Geometry: final body of the model. Coordinates: model frame, mm. Round coordinates to 2 decimals unless told otherwise and drop trailing zeros. Order: outer loops, then holes, each group sorted by start corner. A loop starts at its lowest first (then second) coordinate and runs counter-clockwise, first axis right, second up. Notation, with made-up numbers: (89, 33.25) - (127, 33.25) arc R7 cw to (127, 37.25) - close; hole circle Ø2 at (69.25, 2.25). An arc over 180 degrees is marked (long way). Put each result on its own line as item: value. Start each with the question number.
(1) Section C-C (x = -66). Output: boundary loops of the cut face in (y, z), and give its area (3 significant figures).
(2) Pin query (flat end, axial travel): P1, Ø23.5, axis at x = -187.38, y = 187.38, coming from the +Z side. Return the tip coordinate at first contact, or that it passes through.
(3) Material intervals for L1, parallel to X at y = -196, z = 0.5; L2, parallel to X at y = -91.5, z = 0.1; L3, parallel to Y at x = -7.5, z = 1.6, sorted ascending. Write a range as [from, to].
(4) Section A-A (y = 0). Output: boundary loops of the cut face in (x, z).
(5) Section D-D (y = 70). Output: boundary loops of the cut face in (x, z).
Autodesk Inventor part; units mm, degrees
ref_plane "YZ Plane" through (0, 0, 0) normal (1, 0, 0) x (0, 1, 0)
ref_plane "XZ Plane" through (0, 0, 0) normal (0, 1, 0) x (-1, 0, 0)
ref_plane "XY Plane" through (0, 0, 0) normal (0, 0, 1) x (1, 0, 0)
sketch "Эскиз1" plane through (0, 0, 0) normal (0, 0, 1) x (1, 0, 0)
  circle A0 centre (0, 0) radius 240
  circle A1 centre (0, 0) radius 290
  dimension "d0" = 480
  dimension "d1" = 580
extrude "Выдавливание1" add sketch "Эскиз1" along normal blind 2
sketch "Эскиз2" plane through (0, 0, 2) normal (0, 0, 1) x (1, 0, 0)
  circle A0 centre (0, 0) radius 290
  line L0 (0, 290) -> (0, 265)
  dimension "d4" = 25
hole "Отверстие1" at (0, 265, 2) direction (0, 0, -1) diameter 26 end through all
pattern_circular "Круговой массив1" count 16 over 360 about axis through (0, 0, -10) along (0, 0, 1) of "Отверстие1"
properties part number "Прокладка крышек цилиндра"
Checks:
1. outline: (-282.39, 0) - (-230.75, 0) - (-230.75, 2) - (-282.39, 2) - close; (230.75, 0) - (282.39, 0) - (282.39, 2) - (230.75, 2) - close
1. area: 207 mm²
2. P1: passes through
3. L1: x = [-213.74, -197.12], [-177.65, -138.51], [138.51, 177.65], [197.12, 213.74]
3. L2: x = [-275.19, -253.24], [-236.42, -221.87], [221.87, 236.42], [253.24, 275.19]
3. L3: y = [-289.9, -275.62], [-254.38, -239.88], [239.88, 254.38], [275.62, 289.9]
4. outline: (-290, 0) - (-278, 0) - (-278, 2) - (-290, 2) - close; (-252, 0) - (-240, 0) - (-240, 2) - (-252, 2) - close; (240, 0) - (252, 0) - (252, 2) - (240, 2) - close; (278, 0) - (290, 0) - (290, 2) - (278, 2) - close
5. outline: (-281.42, 0) - (-229.56, 0) - (-229.56, 2) - (-281.42, 2) - close; (229.56, 0) - (281.42, 0) - (281.42, 2) - (229.56, 2) - close
